Answer from the drawing. Dimensions are ordinates in mm from the lowest x, y and z of the part. A direction names the side the tool comes from. Coordinates: 2 decimals unless noted, no trailing zeros. Write each loop counter-clockwise with the first axis right and the second up, starting at its lowest first coordinate (ties: lowest second). Pieces come first, ordered by that corner, then holes.
(1) The mould has two halves that part along Z. Classify the marked faces 1, 2 and 3: +Z half, -Z half, draft (parallel to the pull), parting line (faces both ways), or undercut.
(2) Which of the six approach directions +Z, -Z, +X, -X, +Y, -Y give full straight-line access (tool end or side, diameter ignored) to the marked faces 4, 5 and 6?
(3) Section B-B on y = 7.5 is taken. Write down the section's boundary in (x, z).
(4) Find the intervals of material crossed by probe 1 along Y at (x, z) = (11, 50); probe 2 along X at (y, z) = (31, 75.5), in increasing order.
(5) Given pin 1 (9.5 mm diameter, centred on y = 50, z = 43.5, fed in from +X); pin 2 (4 mm diameter, centred on x = 34, z = 75.5, fed in from +Y); pin 3 (12 mm diameter, centred on y = 7, z = 60, fed in from +X); pin 4 (8 mm diameter, centred on x = 21, y = 82, fed in from +Z), each flat-ended and moving along its own axis, determine where each tip first touches the part or whether it passes through.
(6) Section C-C on z = 25 is taken. Write down the section's boundary in (x, y).
(7) Section D-D on x = 39 is taken. Write down the section's boundary in (y, z).
(8) Section A-A on z = 50 is taken. Write down the section's boundary in (x, y), then the cut area to 3 significant figures.
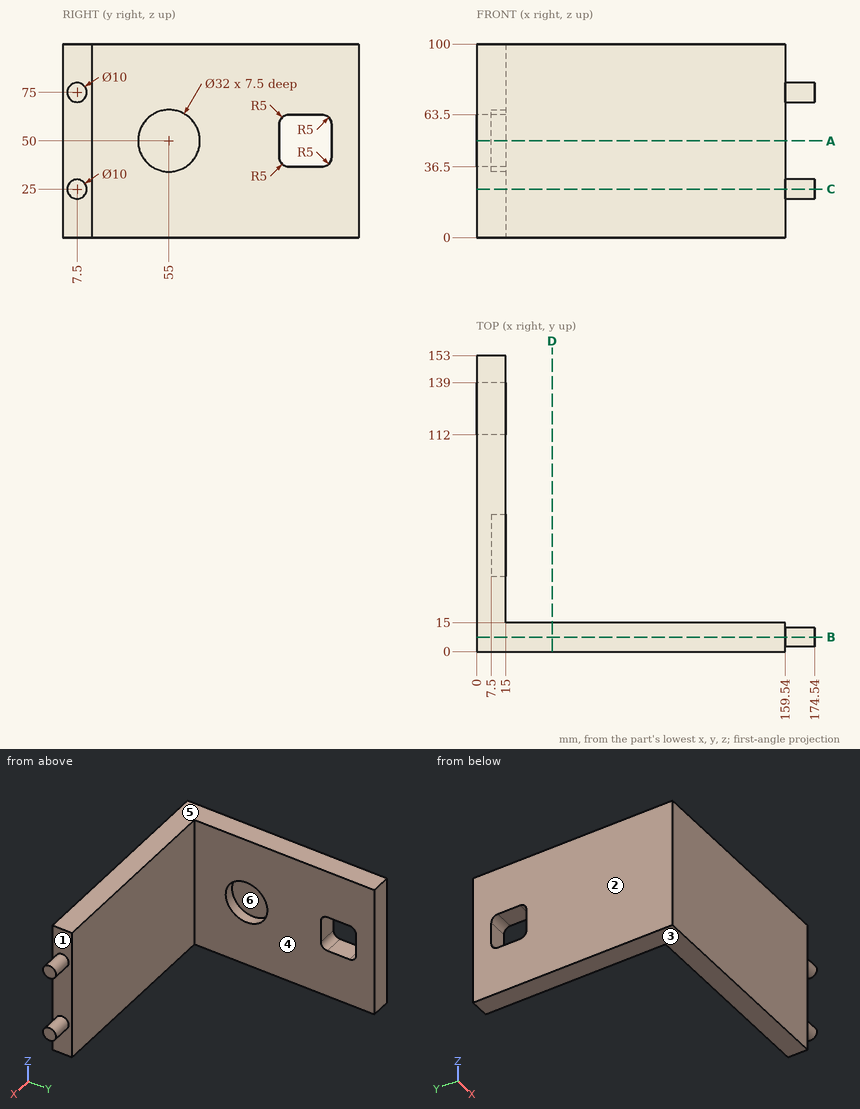
Response:
1. face 1: undercut
1. face 2: draft
1. face 3: -Z half
2. face 4: +Z, -Z, +X, +Y
2. face 5: +Z, +X, -X, +Y, -Y
2. face 6: +X
3. outline: (0, 0) - (159.54, 0) - (159.54, 20) - (174.54, 20) - (174.54, 30) - (159.54, 30) - (159.54, 70) - (174.54, 70) - (174.54, 80) - (159.54, 80) - (159.54, 100) - (0, 100) - close
4. probe 1: y = 0 to 39, 71 to 112, 139 to 153
4. probe 2: x = 0 to 15
5. pin 1: stops at x = 7.5
5. pin 2: stops at y = 15
5. pin 3: stops at x = 159.54
5. pin 4: passes through
6. outline: (0, 0) - (159.54, 0) - (159.54, 2.5) - (174.54, 2.5) - (174.54, 12.5) - (159.54, 12.5) - (159.54, 15) - (15, 15) - (15, 153) - (0, 153) - close
7. outline: (0, 0) - (15, 0) - (15, 100) - (0, 100) - close
8. outline: (0, 0) - (159.54, 0) - (159.54, 15) - (15, 15) - (15, 39) - (7.5, 39) - (7.5, 71) - (15, 71) - (15, 112) - (0, 112) - close; (0, 139) - (15, 139) - (15, 153) - (0, 153) - close
8. area: 3,820 mm2
